The listing builds one solid part. Answer for the finished solid, in the listing's coordinates (mm). Face numbers are marked on the shaded views. A direction names the side the tool comes from. Give positions to 0.01 mm unless a question says otherwise; leave off trailing zeros. Order: outer loops, then holes, each group sorted by start corner. A loop starts at its lowest first (then second) coordinate and runs counter-clockwise, first axis right, second up. Notation, with made-up numbers: (47, -22.5) -> (76, -22.5) arc R21 ccw to (76, -9.5) -> close; hole circle Ø4 at (-37.75, 86). An arc over 180 degrees is marked (long way). One line per question, with ' | ' between items. Start each with the question number.
```python
from build123d import *

# Parameters (mm, degrees)
F0_W     = 300
F0_H     = 195
F1_DEPTH = 60
F3_DEPTH = 180
F7_DEPTH = 121.842539816


with BuildPart() as f1:
    # F0 (on Right) → F1 (new body, symmetric)
    with BuildSketch(Plane.YZ):
        with Locations((-20, -97.5)):
            Rectangle(F0_W, F0_H)
    extrude(amount=F1_DEPTH, both=True)

    # F2 (on face) → F3 (cut)
    with BuildSketch(Plane(origin=(0, 130, 0), x_dir=(-1, 0, 0), z_dir=(0, 1, 0))):
        Polygon((60, -145), (10, -195), (60, -195), align=None)
    extrude(amount=-F3_DEPTH, mode=Mode.SUBTRACT)

    # F6 (on 3pt) → F7 (cut, through all)
    with BuildSketch(Plane(origin=(-60.618556701, 50.5154639175, -60.618556701), x_dir=(0.7930107057, 0.3900052651, -0.4680063181), z_dir=(-0.6092076991, 0.5076730826, -0.6092076991))):
        Polygon((0.7800105302, 209.3402986903), (0.7800105302, 131.2378019312), (63.8308617224, 163.2470219144), align=None)
    extrude(amount=F7_DEPTH, mode=Mode.SUBTRACT)


solid = f1.part
```
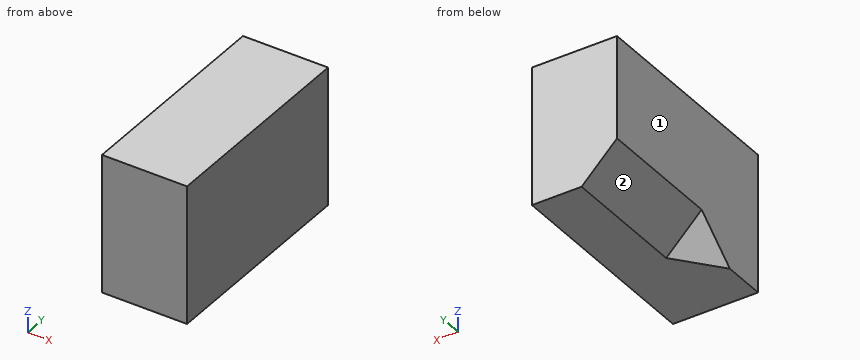
(1) The part is cut by section B-B on y = -54.5. Determine the outline of the cut face in (x, z), plus the area to 3 significant figures.
(2) Consider line 1 (Z direction, x = -33, y = 38); line 2 (X direction, y = -14, z = -162); line 3 (Z direction, x = -38.5, y = 113). Determine where each line is inside the solid, lowest interval first.
(3) The part is cut by section D-D on y = 86. Determine the outline of the cut face in (x, z).
(4) For the marked faces 1 and 2, determine the directions among +Z, -Z, +X, -X, +Y, -Y from which every point of the face is accessible in a straight line to the end or side of a thin tool.
(5) Given P1, Ø1.5, axis at x = 11.5, y = -50.5, coming from the +Z side; P2, Ø5, axis at y = -21.5, z = -153.5, coming from the -X side, each flat-ended and moving along its own axis, determine where each tip first touches the part or whether it passes through.
(6) The part is cut by section A-A on x = -45.5. Determine the outline of the cut face in (y, z).
(7) The part is cut by section C-C on z = -168. Determine the outline of the cut face in (x, y).
Result sheet:
1) outline: (-60, -148.75) -> (-13.75, -195) -> (60, -195) -> (60, 0) -> (-60, 0) -> close | area: 22,300 mm^2
2) line 1: z = -172 to 0 | line 2: x = -43 to 60 | line 3: z = -166.5 to 0
3) outline: (-60, -145) -> (-10, -195) -> (60, -195) -> (60, 0) -> (-60, 0) -> close
4) face 1: +Z, -Z, -X, +Y, -Y | face 2: -Z, -X, +Y
5) P1: stops at z = 0 | P2: stops at x = -54
6) outline: (-170, -195) -> (-92.6, -195) -> (-50, -159.5) -> (130, -159.5) -> (130, 0) -> (-170, 0) -> close
7) outline: (-60, -170) -> (60, -170) -> (60, 130) -> (-37, 130) -> (-37, -50) -> (-60, -77.6) -> close
